```python
from build123d import *

# Parameters (mm, degrees)
ESQUISSE1_W             = 25
ESQUISSE1_H             = 16
ESQUISSE1_W_2           = 60
ESQUISSE1_H_2           = 25
BOSS_EXTRU_1_DEPTH      = 5
CONG_1_R                = 2.5
CONG_2_R                = 4
CONG_3_R                = 5
D_GAGEMENT_M61_D        = 6.6
D_GAGEMENT_M201_D       = 21
ENL_V_MAT_EXTRU_1_REACH = 220.607
ESQUISSE11_R            = 4.25
BOSS_EXTRU_2_DEPTH      = 5
D_GAGEMENT_M62_D        = 6.6
D_GAGEMENT_M62_DEPTH    = 5
D_GAGEMENT_M62_TIP      = 1.982840043
CONG_4_R                = 5
TROU_TARAUD_M4X0_71_D   = 3.3
CHANFREIN1_SIZE         = 3


with BuildPart() as part:
    # Esquisse1 → Boss.-Extru.1 (new body)
    with BuildSketch(Plane.XY):
        Polygon((0, 0), (0, -52), (55, -52), (55, -96), (80, -96), (80, -108), (110, -108), (110, -96), (135, -96), (135, -52), (190, -52), (190, 0), align=None)
        with Locations((95, -31)):
            Rectangle(ESQUISSE1_W, ESQUISSE1_H, mode=Mode.SUBTRACT)
        with Locations((95, -67.5)):
            Rectangle(ESQUISSE1_W_2, ESQUISSE1_H_2, mode=Mode.SUBTRACT)
        with BuildLine():
            Line((76, -6.71), (114, -6.71))
            ThreePointArc((114, -6.71), (118, -10.71), (114, -14.71))
            Line((114, -14.71), (76, -14.71))
            ThreePointArc((76, -14.71), (72, -10.71), (76, -6.71))
        make_face(mode=Mode.SUBTRACT)
    extrude(amount=BOSS_EXTRU_1_DEPTH)

    # Congé1
    cong_1_edges = [part.edges().sort_by_distance(p)[0] for p in [
        (82.5, -23, 2.5),
        (82.5, -39, 2.5),
        (107.5, -39, 2.5),
        (107.5, -23, 2.5),
    ]]
    fillet(cong_1_edges, radius=CONG_1_R)

    # Congé2
    cong_2_edges = [part.edges().sort_by_distance(p)[0] for p in [
        (65, -55, 2.5),
        (65, -80, 2.5),
        (125, -80, 2.5),
        (125, -55, 2.5),
    ]]
    fillet(cong_2_edges, radius=CONG_2_R)

    # Congé3
    cong_3_edges = [part.edges().sort_by_distance(p)[0] for p in [
        (135, -52, 2.5),
        (55, -52, 2.5),
    ]]
    fillet(cong_3_edges, radius=CONG_3_R)

    # Dégagement M61 (through all)
    with Locations(Plane.XY.offset(5)):
        with Locations((10, -10), (180, -10)):
            Hole(D_GAGEMENT_M61_D / 2)

    # Dégagement M201 (through all)
    with Locations(Plane.XY.offset(5)):
        with Locations((32, -14), (158, -14)):
            Hole(D_GAGEMENT_M201_D / 2)

    # Esquisse11 → Enlèv. mat.-Extru.1 (cut, up to next)
    with BuildSketch(Plane.XY.offset(5), mode=Mode.PRIVATE) as enl_v_mat_extru_1_sk1:
        with Locations((54.5, -11.5)):
            Circle(ESQUISSE11_R)
    enl_v_mat_extru_1_tool1 = extrude(enl_v_mat_extru_1_sk1.sketch, amount=-ENL_V_MAT_EXTRU_1_REACH, mode=Mode.PRIVATE) & part.part
    # Esquisse11 → Enlèv. mat.-Extru.1 (cut, up to next)
    with BuildSketch(Plane.XY.offset(5), mode=Mode.PRIVATE) as enl_v_mat_extru_1_sk2:
        with Locations((135.5, -11.5)):
            Circle(ESQUISSE11_R)
    enl_v_mat_extru_1_tool2 = extrude(enl_v_mat_extru_1_sk2.sketch, amount=-ENL_V_MAT_EXTRU_1_REACH, mode=Mode.PRIVATE) & part.part
    add(enl_v_mat_extru_1_tool1.solids().sort_by_distance((54.5, -11.5, 5))[0], mode=Mode.SUBTRACT)
    add(enl_v_mat_extru_1_tool2.solids().sort_by_distance((135.5, -11.5, 5))[0], mode=Mode.SUBTRACT)

    # Esquisse13 → Boss.-Extru.2 (add)
    with BuildSketch(Plane.XY.offset(5)):
        Polygon((0, 0), (-27, -27), (-27, -52), (0, -52), align=None)
        Polygon((217, -52), (190, -52), (190, 0), (217, -27), align=None)
    extrude(amount=-BOSS_EXTRU_2_DEPTH)

    # Dégagement M62
    with Locations(Plane.XY.offset(5)):
        with Locations((65, -44), (125, -44), (125, -85), (65, -85)):
            Hole(D_GAGEMENT_M62_D / 2, depth=D_GAGEMENT_M62_DEPTH)
            with Locations((0, 0, -(D_GAGEMENT_M62_DEPTH + D_GAGEMENT_M62_TIP / 2))):  # 118° drill point
                Cone(0, D_GAGEMENT_M62_D / 2, D_GAGEMENT_M62_TIP, mode=Mode.SUBTRACT)

    # Congé4
    cong_4_edges = [part.edges().sort_by_distance(p)[0] for p in [
        (110, -96, 2.5),
        (80, -96, 2.5),
    ]]
    fillet(cong_4_edges, radius=CONG_4_R)

    # Trou taraudé M4x0.71 (through all)
    with Locations(Plane.XY.offset(5)):
        with Locations((88, -103), (102, -103)):
            Hole(TROU_TARAUD_M4X0_71_D / 2)

    # Chanfrein1
    # the kernel refuses this chamfer: 3 mm, written as the material it takes off along each edge
    with BuildSketch(Plane(origin=(180, -10, 5), x_dir=(-1, 0, 0), z_dir=(0, -1, 0))) as chanfrein1_piece_1:
        Polygon((3.3, CHANFREIN1_SIZE), (3.3 + CHANFREIN1_SIZE, 0), (3.3, 0), align=None)
    revolve(axis=Axis((180, -10, 5), (0, 0, -1)), mode=Mode.SUBTRACT)
    with BuildSketch(Plane(origin=(10, -10, 5), x_dir=(-1, 0, 0), z_dir=(0, -1, 0))) as chanfrein1_piece_2:
        Polygon((3.3, CHANFREIN1_SIZE), (3.3 + CHANFREIN1_SIZE, 0), (3.3, 0), align=None)
    revolve(axis=Axis((10, -10, 5), (0, 0, -1)), mode=Mode.SUBTRACT)
    with BuildSketch(Plane(origin=(65, -85, 5), x_dir=(-1, 0, 0), z_dir=(0, -1, 0))) as chanfrein1_piece_3:
        Polygon((3.3, CHANFREIN1_SIZE), (3.3 + CHANFREIN1_SIZE, 0), (3.3, 0), align=None)
    revolve(axis=Axis((65, -85, 5), (0, 0, -1)), mode=Mode.SUBTRACT)
    with BuildSketch(Plane(origin=(125, -85, 5), x_dir=(-1, 0, 0), z_dir=(0, -1, 0))) as chanfrein1_piece_4:
        Polygon((3.3, CHANFREIN1_SIZE), (3.3 + CHANFREIN1_SIZE, 0), (3.3, 0), align=None)
    revolve(axis=Axis((125, -85, 5), (0, 0, -1)), mode=Mode.SUBTRACT)
    with BuildSketch(Plane(origin=(125, -44, 5), x_dir=(-1, 0, 0), z_dir=(0, -1, 0))) as chanfrein1_piece_5:
        Polygon((3.3, CHANFREIN1_SIZE), (3.3 + CHANFREIN1_SIZE, 0), (3.3, 0), align=None)
    revolve(axis=Axis((125, -44, 5), (0, 0, -1)), mode=Mode.SUBTRACT)
    with BuildSketch(Plane(origin=(65, -44, 5), x_dir=(-1, 0, 0), z_dir=(0, -1, 0))) as chanfrein1_piece_6:
        Polygon((3.3, CHANFREIN1_SIZE), (3.3 + CHANFREIN1_SIZE, 0), (3.3, 0), align=None)
    revolve(axis=Axis((65, -44, 5), (0, 0, -1)), mode=Mode.SUBTRACT)


solid = part.part
```
Can you work these out from the model? Positions are in its coordinate system, mm. A direction names the side the tool comes from. Give positions to 0.01 mm unless a question says otherwise; leave off trailing zeros. Order: outer loops, then holes, each group sorted by start corner. A loop starts at its lowest first (then second) coordinate and runs counter-clockwise, first axis right, second up. Notation, with made-up numbers: M -24,66 L 8,66 A27 cw 8,91 Z; hole C 6,32.25 d4. An arc over 180 degrees is marked long. Write item = value, one per line. Start each with the question number.
Q1. Suppose I cut it at D-D (z = 3.25). Count the separate pieces of the cut face and the enclosed holes in it, plus the area to 3 significant figures.
Q2. We'd pull the mould along Y, two halves only. Please class faces 1 (the flat face through (178, -52, 2)), 2 (the conical face through (123.391, -47.094, 2.188)), 3 (the flat face through (-27, -39, 3)), 4 (the flat face through (-13, -13, 3)): pulls with the +Y half, pulls with the -Y half, needs draft (parallel to the pull), parting line crosses it, or undercut.
Q3. For faces 5 (the flat face through (82.5, -31, 2)), 6 (the conical face through (67.8, -46.1, 2.2)), which set-ups out of +Z, -Z, +X, -X, +Y, -Y let a thin tool reach every point of the face, with its end or its side?
Q4. I need wall thicknesses on probe 1 along X at (y, z) = (-72.5, 1.25); probe 2 along Y at (x, z) = (102, 1.95); probe 3 along Y at (x, z) = (120, 2.9). Which ranges of each line are inside material? Lowest first, please. Write a range as [from, to].
Q5. Will these pins go through, and if not, where does the flat tip stop? pin 1 Ø10.5 at (x, y) = (65, -85) entering from +Z; pin 2 Ø2.5 at (y, z) = (-66.5, 1.5) entering from +X; pin 3 Ø1.5 at (y, z) = (-106, 3.5) entering from +X.
Q6. Suppose I cut it at B-B (x = 32). Write out the boundary of the cut face in (y, z), plus the area to 3 significant figures.
Q7. Suppose I cut it at A-A (y = -44). Write out the boundary of the cut face in (x, z).
Q8. Suppose I cut it at C-C (y = -66). Write out the boundary of the cut face in (x, z), plus the area to 4 significant figures.
Check result:
q1.separate_pieces = 1
q1.enclosed_holes = 15
q1.area = 12,400 mm2
q2.face_1 = pulls with the -Y half
q2.face_2 = undercut
q2.face_3 = needs draft
q2.face_4 = pulls with the +Y half
q3.face_5 = +Z, -Z
q3.face_6 = +Z
q4.probe_1 = [55, 65], [125, 135]
q4.probe_2 = [-108, -104.65], [-101.35, -80], [-55, -39], [-23, -14.71], [-6.71, 0]
q4.probe_3 = [-96, -80], [-55, 0]
q5.pin_1 = 3.95
q5.pin_2 = 135
q5.pin_3 = 110
q6.outline = M -52,0 L -24.5,0 L -24.5,5 L -52,5 Z; M -3.5,0 L 0,0 L 0,5 L -3.5,5 Z
q6.area = 155 mm2
q7.outline = M -27,0 L 61.7,0 L 61.7,2 L 58.7,5 L -27,5 Z; M 68.3,0 L 121.7,0 L 121.7,2 L 118.7,5 L 71.3,5 L 68.3,2 Z; M 128.3,0 L 217,0 L 217,5 L 131.3,5 L 128.3,2 Z
q8.outline = M 55,0 L 65,0 L 65,5 L 55,5 Z; M 125,0 L 135,0 L 135,5 L 125,5 Z
q8.area = 100.0 mm2
